from build123d import *

# Parameters (mm, degrees)
SKETCH1_W           = 41.91
SKETCH1_H           = 15.875
BOSS_EXTRUDE1_DEPTH = 12.7
SKETCH2_W           = 12.7
SKETCH2_H           = 9.525
CUT_EXTRUDE1_DEPTH  = 46.263519803
CUT_EXTRUDE2_DEPTH  = 28.045335088
HOLE1_D             = 5.1054
HOLE1_DEPTH         = 12.7
FILLET1_R           = 5.08


with BuildPart() as part:
    # Sketch1 → Boss-Extrude1 (new body)
    with BuildSketch(Plane(origin=(0, 6.35, 0), x_dir=(1, 0, 0), z_dir=(0, 1, 0))):
        with Locations((0, 7.9375)):
            Rectangle(SKETCH1_W, SKETCH1_H)
    extrude(amount=-BOSS_EXTRUDE1_DEPTH)

    # Sketch2 → Cut-Extrude1 (cut, through all)
    with BuildSketch(Plane(origin=(20.955, 0, 0), x_dir=(0, 0, -1), z_dir=(1, 0, 0))):
        with Locations((9.525, 1.5875)):
            Rectangle(SKETCH2_W, SKETCH2_H)
    extrude(amount=-CUT_EXTRUDE1_DEPTH, mode=Mode.SUBTRACT)

    # Sketch3 → Cut-Extrude2 (cut, through all)
    with BuildSketch(Plane.XY):
        with BuildLine():
            Line((-13.843, -2.54), (10.033, -2.54))
            ThreePointArc((10.033, -2.54), (12.573, 0), (10.033, 2.54))
            Line((10.033, 2.54), (-13.843, 2.54))
            ThreePointArc((-13.843, 2.54), (-16.383, 0), (-13.843, -2.54))
        make_face()
    extrude(amount=-CUT_EXTRUDE2_DEPTH, mode=Mode.SUBTRACT)

    # Hole1
    with Locations(Plane(origin=(0, -6.35, 0), x_dir=(-1, 0, 0), z_dir=(0, -1, 0))):
        with Locations((10.795, 10.16), (-14.605, 10.16)):
            Hole(HOLE1_D / 2, depth=HOLE1_DEPTH)

    # Fillet1
    fillet1_edges = [part.edges().sort_by_distance(p)[0] for p in [
        (-20.955, 6.35, -1.5875),
        (20.955, 6.35, -1.5875),
        (-20.955, -4.7625, -15.875),
        (20.955, -4.7625, -15.875),
    ]]
    fillet(fillet1_edges, radius=FILLET1_R)


solid = part.part
The listing builds one solid part. Answer for the finished solid, in the listing's coordinates (mm). A direction names the side the tool comes from. Give positions to 0.01 mm unless a question says otherwise; leave off trailing zeros. Order: outer loops, then holes, each group sorted by start corner. A loop starts at its lowest first (then second) coordinate and runs counter-clockwise, first axis right, second up. Notation, with made-up numbers: (-35, 63) - (-17, 63) arc R32 ccw to (-17, 99) - close; hole circle Ø7 at (13.5, 87). An arc over 180 degrees is marked (long way). One line per item, written item: value. Start each with the question number.
1) A cutting plane is placed at C-C on x = -1.5. Give the vertices of the cut face in (y, z) (3 decimals), then the cut area to 3 significant figures.
2) A cutting plane is placed at A-A on y = -4.5. Give the vertices of the cut face in (x, z) (3 decimals).
3) The mould has two halves that part along X. Classify faces 4 (the face through (-20.955, -3.33, -4.12)), 5 (the face through (15.783, -4.74, -7.895)), 6 (the face through (0, -6.35, -8)), 7 (the face through (-9.617, -4.74, -7.895)): released by +X, released by -X, zero draft, split by the parting line, or undercut.
4) Given pin 1 Ø3 at (x, z) = (15.5, -12.5) entering from -Y; pin 2 Ø1 at (x, y) = (0.5, 0.5) entering from +Z; pin 3 Ø3 at (x, z) = (-5.5, -10) entering from +Y (3 decimals), each flat-ended and moving along its own axis, determine where each tip first touches the part or whether it passes through.
5) A tool of negligible diameter and unlimited length cuts with its end or side. For faces 1 (the face through (0, -3.175, -9)), 2 (the face through (-2, -2.54, -2)), 3 (the face through (0, -3, 0)), from which of +Z, -Z, +X, -X, +Y, -Y can it reach the whole face along a straight path? Write none if from no direction.
6) A cutting plane is placed at D-D on y = 0. Give the vertices of the cut face in (x, z) (3 decimals).
7) Find the intervals of material crossed by L1, parallel to X at y = -5.35, z = -10.16 (3 decimals); L2, parallel to Y at x = 19, z = -11.5 (3 decimals); L3, parallel to Z at x = 8.5, y = 3.5 (3 decimals), in increasing order.
8) A cutting plane is placed at B-B on z = -10.16. Give the vertices of the cut face in (x, y) (3 decimals), then the cut area to 3 significant figures.
Answer sheet:
1. outline: (-6.35, -15.875) - (-3.175, -15.875) - (-3.175, -3.175) - (-2.54, -3.175) - (-2.54, 0) - (-6.35, 0) - close; (2.54, -3.175) - (6.35, -3.175) - (6.35, 0) - (2.54, 0) - close
1. area: 64.5 mm2
2. outline: (-20.955, -10.795) arc R5.08 ccw to (-15.875, -15.875) - (15.875, -15.875) arc R5.08 ccw to (20.955, -10.795) - (20.955, 0) - (-20.955, 0) - close; hole circle Ø5.105 at (-10.795, -10.16); hole circle Ø5.105 at (14.605, -10.16)
3. face 4: released by -X
3. face 5: undercut
3. face 6: zero draft
3. face 7: undercut
4. pin 1: stops at y = -6.35
4. pin 2: passes through
4. pin 3: stops at y = -3.175
5. face 1: -Z, +X, -X, +Y
5. face 2: +Z, -Z
5. face 3: +Z, +X, -X, +Y, -Y
6. outline: (-20.955, -3.175) - (-16.383, -3.175) - (-16.383, 0) - (-20.955, 0) - close; (12.573, -3.175) - (20.955, -3.175) - (20.955, 0) - (12.573, 0) - close
7. L1: x = -20.955 to -13.348, -8.242 to 12.052, 17.158 to 20.955
7. L2: y = -6.35 to -3.175
7. L3: z = -3.175 to 0
8. outline: (-20.955, -6.35) - (-13.348, -6.35) - (-13.348, -3.175) - (-20.955, -3.175) - close; (-8.242, -6.35) - (12.052, -6.35) - (12.052, -3.175) - (-8.242, -3.175) - close; (17.158, -6.35) - (20.955, -6.35) - (20.955, -3.175) - (17.158, -3.175) - close
8. area: 101 mm2
